Design review of the part built by this model. Coordinates are the model's own, in mm. Face numbers are marked on the shaded views. A direction names the side the tool comes from. Coordinates: 2 decimals unless noted, no trailing zeros. Write each loop counter-clockwise with the first axis right and the second up, starting at its lowest first coordinate (ties: lowest second). Pieces come first, ordered by that corner, then holes.
Q1. The part is to be moulded in two halves that separate along Z. For the marked faces 5, 6 and 7, say which applies: released by +Z, released by -Z, zero draft, split by the parting line, or undercut.
Q2. Take a section at B-B, the plane z = -13.5. Write out the cut boundary in (x, y).
Q3. Take a section at A-A, the plane x = 9.75. Write out the cut boundary in (y, z), plus the area to 3 significant figures.
Q4. Take a section at C-C, the plane x = 1. Write out the cut boundary in (y, z), plus the area to 3 significant figures.
Q5. For L1, parallel to Y at x = 5.75, z = -22; L2, parallel to Z at x = 10, y = 15.5; L3, parallel to Y at x = 6, z = -20.5, list the stretches that pass through material, from the lowest coordinate up.
Q6. For pin 1 Ø0.6 at (y, z) = (-4.5, -5) entering from -X; pin 2 Ø6 at (x, y) = (5, 14) entering from +Z; pin 3 Ø1.7 at (x, y) = (6.205, -2.415) entering from +Z (3 decimals); pin 4 Ø6 at (x, z) = (7, 0.5) entering from -Y, all flat-tipped, find the tip position at first contact; note any pin that passes through.
Q7. For the marked faces 1, 2, 3 and 4, list the 3-axis set-ups (+Z, -Z, +X, -X, +Y, -Y) from which the entire face can be reached by the end or side of a thin tool; tool diameter is ignored.
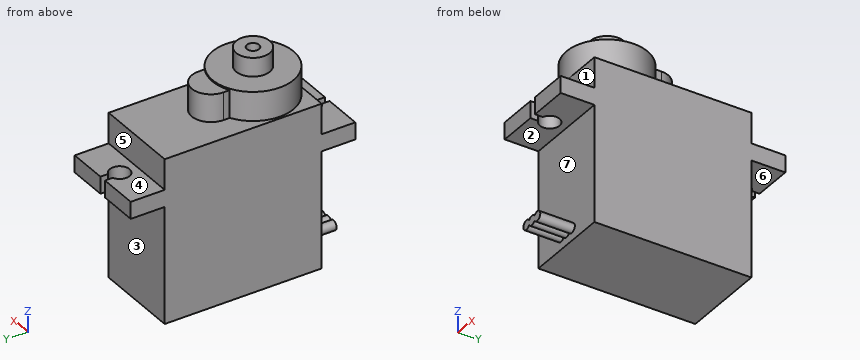
from build123d import *

# Parameters (mm, degrees)
SKETCH1_W                = 12.41
SKETCH1_H                = 23.75
BOSS_EXTRUDE1_DEPTH      = 22.71
SKETCH2_R                = 5.875
BOSS_EXTRUDE3_DEPTH      = 4.2
BOSS_EXTRUDE4_DEPTH      = 4
BOSS_EXTRUDE5_DEPTH      = 4.87
BOSS_EXTRUDE5_DEPTH_BACK = 27.62
SKETCH6_W                = 12.41
SKETCH6_H                = 2.46
SKETCH8_R                = 1.43
CUT_EXTRUDE1_DEPTH       = 36.929209565
SKETCH9_W                = 1.02
SKETCH9_H                = 2.455
CUT_EXTRUDE2_DEPTH       = 36.929209565
SKETCH10_R               = 2.45
SKETCH10_R_2             = 0.885
BOSS_EXTRUDE7_DEPTH      = 2.7
BOSS_EXTRUDE8_DEPTH      = 5


with BuildPart() as part:
    # Sketch1 → Boss-Extrude1 (new body)
    with BuildSketch(Plane(origin=(0, 0, 0), x_dir=(1, 0, 0), z_dir=(0, 1, 0))):
        with Locations((6.205, 11.875)):
            Rectangle(SKETCH1_W, SKETCH1_H)
    extrude(amount=BOSS_EXTRUDE1_DEPTH)

    # Sketch2 → Boss-Extrude3 (add)
    with BuildSketch(Plane.XY):
        with Locations(Location((6.205, 5.875, 0), (0, 0, 270))):
            Circle(SKETCH2_R)
    extrude(amount=BOSS_EXTRUDE3_DEPTH)

    # Sketch4 → Boss-Extrude4 (add)
    with BuildSketch(Plane.XY):
        with BuildLine():
            Line((3.43, 11.965), (3.43, 11.053320191))
            Line((3.43, 11.053320191), (8.98, 11.053320191))
            Line((8.98, 11.053320191), (8.98, 11.965))
            ThreePointArc((8.98, 11.965), (6.205, 14.74), (3.43, 11.965))
        make_face()
    extrude(amount=BOSS_EXTRUDE4_DEPTH)

    # Sketch6 → Boss-Extrude5 (add, two sides: drawn at the far end of the back side and taken through both)
    with BuildSketch(Plane.XZ.offset(-BOSS_EXTRUDE5_DEPTH_BACK)):
        with Locations((6.205, -5.64)):
            Rectangle(SKETCH6_W, SKETCH6_H)
    extrude(amount=BOSS_EXTRUDE5_DEPTH + BOSS_EXTRUDE5_DEPTH_BACK)

    # Sketch8 → Cut-Extrude1 (cut, through all)
    with BuildSketch(Plane.XY.offset(-4.41)):
        with Locations((6.205, 25.165)):
            Circle(SKETCH8_R)
        with Locations((6.205, -2.415)):
            Circle(SKETCH8_R)
    extrude(amount=-CUT_EXTRUDE1_DEPTH, mode=Mode.SUBTRACT)

    # Sketch9 → Cut-Extrude2 (cut, through all)
    with BuildSketch(Plane.XY.offset(-4.41)):
        with Locations((6.205, 26.3925)):
            Rectangle(SKETCH9_W, SKETCH9_H)
        with Locations((6.205, -3.6425)):
            Rectangle(SKETCH9_W, SKETCH9_H)
    extrude(amount=-CUT_EXTRUDE2_DEPTH, mode=Mode.SUBTRACT)

    # Sketch10 → Boss-Extrude7 (add)
    with BuildSketch(Plane.XY.offset(4.2)):
        with Locations(Location((6.205, 5.875, 0), (0, 0, 180))):
            Circle(SKETCH10_R)
        with Locations(Location((6.205, 5.875, 0), (0, 0, 180))):
            Circle(SKETCH10_R_2, mode=Mode.SUBTRACT)
    extrude(amount=BOSS_EXTRUDE7_DEPTH)

    # Sketch12 → Boss-Extrude8 (add)
    with BuildSketch(Plane.XZ):
        with BuildLine():
            ThreePointArc((5.61, -22.289411255), (6.205, -22.635), (6.8, -22.289411255))
            ThreePointArc((6.8, -22.289411255), (8.08, -21.95), (6.8, -21.610588745))
            ThreePointArc((6.8, -21.610588745), (6.205, -21.265), (5.61, -21.610588745))
            ThreePointArc((5.61, -21.610588745), (4.33, -21.95), (5.61, -22.289411255))
        make_face()
    extrude(amount=BOSS_EXTRUDE8_DEPTH)


solid = part.part
Responses:
1. face 5: zero draft
1. face 6: released by -Z
1. face 7: undercut
2. outline: (0, 0) - (12.41, 0) - (12.41, 22.71) - (0, 22.71) - close
3. outline: (-4.87, -6.87) - (0, -6.87) - (0, -23.75) - (22.71, -23.75) - (22.71, -6.87) - (27.62, -6.87) - (27.62, -4.41) - (22.71, -4.41) - (22.71, 0) - (10.56, 0) - (10.56, 4.2) - (1.19, 4.2) - (1.19, 0) - (0, 0) - (0, -4.41) - (-4.87, -4.41) - close
3. area: 603 mm2
4. outline: (-4.87, -6.87) - (0, -6.87) - (0, -23.75) - (22.71, -23.75) - (22.71, -6.87) - (27.62, -6.87) - (27.62, -4.41) - (22.71, -4.41) - (22.71, 0) - (8.6, 0) - (8.6, 4.2) - (3.15, 4.2) - (3.15, 0) - (0, 0) - (0, -4.41) - (-4.87, -4.41) - close
4. area: 586 mm2
5. L1: y = -5 to 22.71
5. L2: z = -23.75 to 0
5. L3: y = 0 to 22.71
6. pin 1: stops at x = 0
6. pin 2: stops at z = 4.2
6. pin 3: stops at z = -21.265
6. pin 4: stops at y = 0
7. face 1: +Z, +X, -X, -Y
7. face 2: +X, -X, -Y
7. face 3: -Z, +X, -X, +Y
7. face 4: +Z, +X, -X, +Y
